Check sheet for the modelled part. Datum: model origin and axes. Units: mm. Face numbers are marked on the shaded views. Give positions to 0.01 mm unless a question says otherwise; leave off trailing zeros. Write each loop counter-clockwise with the first axis right and the second up, starting at its lowest first coordinate (ties: lowest second). Pieces come first, ordered by that corner, then holes. Notation, with made-up numbers: (60.5, 42.25) -> (76.5, 42.25) arc R32 ccw to (76.5, 74.25) -> close; hole circle Ø5 at (28, 68). An arc over 180 degrees is marked (long way). Write each question's results on one line, items separated by ' | '. Start each with the question number.
```python
from build123d import *

# Parameters (mm, degrees)
SKIZZE1_W            = 6
SKIZZE1_H            = 2
M2_GEWINDEBOHRUNG1_D = 1.6
FASE1_SIZE           = 0.5
FASE1_SIZE2          = 0.181985117
FASE2_SIZE           = 1
FASE2_SIZE2          = 0.577350269


with BuildPart() as part:
    # Skizze1 → Rotation1 (revolve)
    with BuildSketch(Plane.XY):
        with Locations((3, 1.5)):
            Rectangle(SKIZZE1_W, SKIZZE1_H)
    revolve(axis=Axis((0, 0, 0), (1, 0, 0)))

    # M2 Gewindebohrung1 (through all)
    with Locations(Plane(origin=(6, 0, 0), x_dir=(0, 0, -1), z_dir=(1, 0, 0))):
        with Locations((0, 0)):
            Hole(M2_GEWINDEBOHRUNG1_D / 2)

    # Fase1
    fase1_edges = [part.edges().sort_by_distance(p)[0] for p in [
        (6, -2.5, 0),
        (0, -2.5, 0),
    ]]
    fase1_side = [part.faces().sort_by_distance(p)[0] for p in [
        (3, -2.5, 0),
    ]]
    chamfer(fase1_edges, length=FASE1_SIZE, length2=FASE1_SIZE2, reference=fase1_side[0])

    # Fase2
    fase2_edges = [part.edges().sort_by_distance(p)[0] for p in [
        (6, 0, -0.8),
        (0, 0, -0.8),
    ]]
    fase2_side = [part.faces().sort_by_distance(p)[0] for p in [
        (3, 0, -0.8),
    ]]
    chamfer(fase2_edges, length=FASE2_SIZE, length2=FASE2_SIZE2, reference=fase2_side[0])


solid = part.part
```
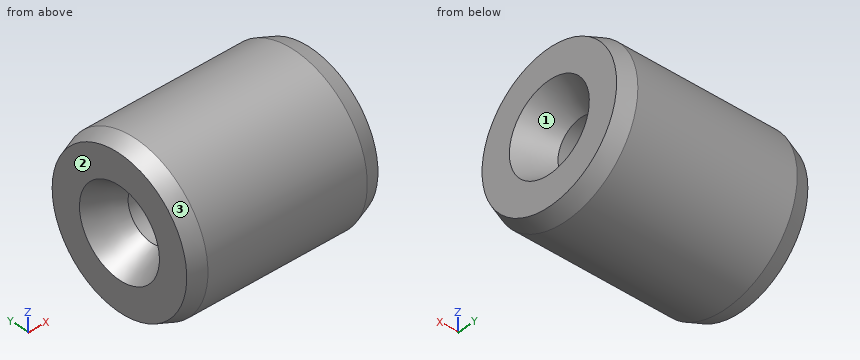
Item 1: Section check D-D on x = 0.85. Record the boundary of the cut face in (y, z), then the cut area to 3 significant figures.
Item 2: Section check C-C on x = 3.1. Record the boundary of the cut face in (y, z).
Item 3: Thickness scan on probe 1 along Y at (x, z) = (3.95, -0.55); probe 2 along Z at (x, y) = (3.65, 0.35); probe 3 along Y at (x, z) = (2.15, 1.7). Record the ranges inside material, lowest first. Write a range as from..to.
Item 4: Depth check by flat-ended pin: pin 1 Ø2 at (x, y) = (1, 2) entering from +Z; pin 2 Ø2 at (x, z) = (2, 2) entering from -Y; pin 3 Ø2 at (x, y) = (1, 1.5) entering from +Z. Enter the tip coordinate at first touch or a pass-through.
Item 5: Mould release check, pull along Y, two halves, no side actions. Record for the marked faces 1, 2 and 3: pulls with the +Y half, pulls with the -Y half, needs draft (parallel to the pull), parting line crosses it, or undercut.
Item 6: Section check A-A on y = 0. Record the boundary of the cut face in (x, z).
Check sheet entries:
1) outline: circle Ø5 at (0, 0); hole circle Ø1.77 at (0, 0) | area: 17.2 mm^2
2) outline: circle Ø5 at (0, 0); hole circle Ø1.6 at (0, 0)
3) probe 1: y = -2.44..-0.58, 0.58..2.44 | probe 2: z = -2.48..-0.72, 0.72..2.48 | probe 3: y = -1.83..1.83
4) pin 1: stops at z = 2.29 | pin 2: stops at y = -2.29 | pin 3: stops at z = 2.45
5) face 1: undercut | face 2: needs draft | face 3: parting line crosses it
6) outline: (0, -2.32) -> (0.5, -2.5) -> (5.5, -2.5) -> (6, -2.32) -> (6, -1.38) -> (5, -0.8) -> (1, -0.8) -> (0, -1.38) -> close; (0, 1.38) -> (1, 0.8) -> (5, 0.8) -> (6, 1.38) -> (6, 2.32) -> (5.5, 2.5) -> (0.5, 2.5) -> (0, 2.32) -> close
